Source: three-view drawing plus pictorial views. Frame: mm from the lowest corner of the part. A direction names the side the tool comes from. Round coordinates to 2 decimals unless told otherwise and drop trailing zeros. Loops run counter-clockwise (first coordinate to the right, second up) from the corner with the lowest first, then second, coordinate; pieces in that order, holes last. Notation, with made-up numbers: (82, 23) -> (116, 23) arc R28 cw to (116, 46) -> close; hole circle Ø8 at (-10, 59.5). An arc over 180 degrees is marked (long way). Return JSON: item names as keys, results as strings. Group by question number.
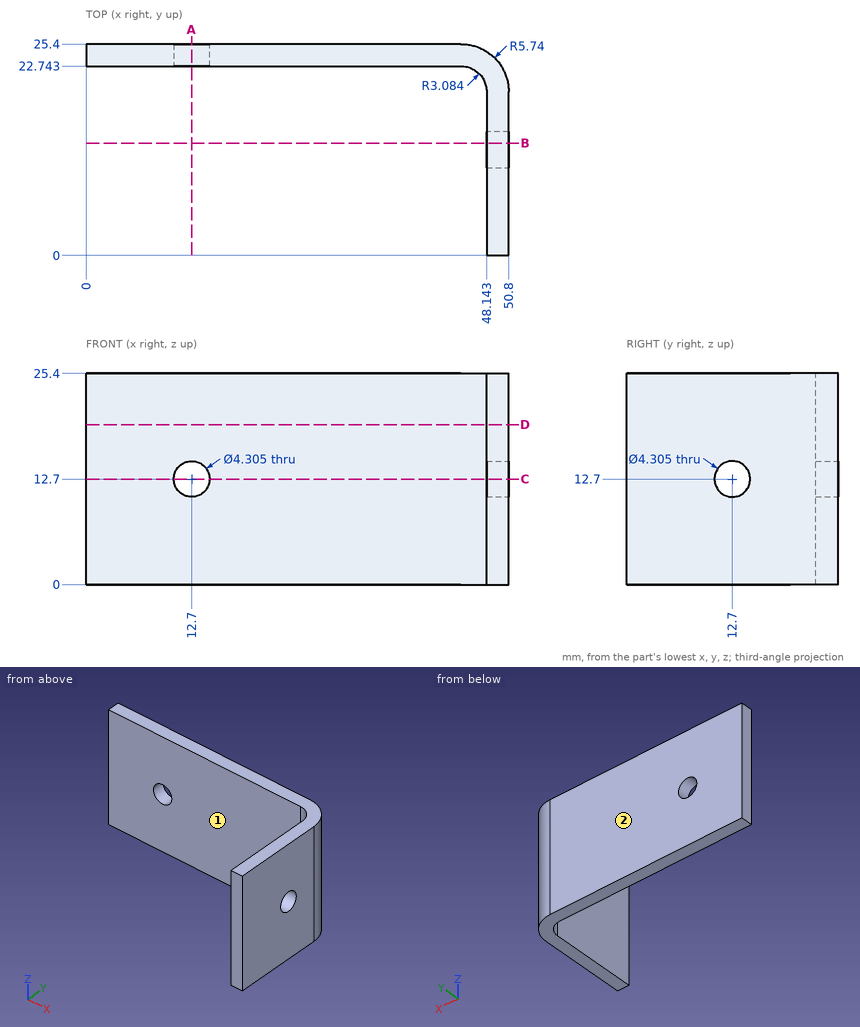
(1) Cut plane A-A (x = 12.7). Return loops of the section in (y, z).
(2) Cut plane C-C (z = 12.7). Return loops of the section in (x, y).
(3) Pin query (flat end, axial travel): pin 1 (5 mm diameter, centred on x = 12.7, z = 12.7, fed in from +Y); pin 2 (12 mm diameter, centred on x = 18, z = 19, fed in from -Y); pin 3 (3 mm diameter, centred on y = 12, z = 13.5, fed in from -X); pin 4 (12 mm diameter, centred on y = 15.5, z = 20, fed in from -X) (1 decimal). Return the tip coordinate at first contact, or that it passes through.
(4) Cut plane B-B (y = 13.5). Return loops of the section in (x, z).
(5) Set-up query: the marked faces 1 and 2. Return all of +Z, -Z, +X, -X, +Y, -Y with unobstructed straight access to the full face (end or side cutting, diameter ignored); none if empty.
(6) Cut plane D-D (z = 19.25). Return loops of the section in (x, y), and give its area (3 significant figures).
(7) Ray query, line 1 (Z direction, x = 49.95, y = 12.7); line 2 (Y direction, x = 15.5, z = 3.25); line 3 (X direction, y = 15.75, z = 23.5). Return the intervals inside material, ascending.
Answers follow:
{
 "1": {"outline": "(22.74, 0) -> (25.4, 0) -> (25.4, 10.55) -> (22.74, 10.55) -> close; (22.74, 14.85) -> (25.4, 14.85) -> (25.4, 25.4) -> (22.74, 25.4) -> close"},
 "2": {"outline": "(0, 22.74) -> (10.55, 22.74) -> (10.55, 25.4) -> (0, 25.4) -> close; (14.85, 22.74) -> (45.06, 22.74) arc R3.08 cw to (48.14, 19.66) -> (48.14, 14.85) -> (50.8, 14.85) -> (50.8, 19.66) arc R5.74 ccw to (45.06, 25.4) -> (14.85, 25.4) -> close; (48.14, 0) -> (50.8, 0) -> (50.8, 10.55) -> (48.14, 10.55) -> close"},
 "3": {"pin 1": "y = 25.4", "pin 2": "y = 22.74", "pin 3": "x = 48.14", "pin 4": "x = 47.5"},
 "4": {"outline": "(48.14, 0) -> (50.8, 0) -> (50.8, 10.7) -> (48.14, 10.7) -> close; (48.14, 14.7) -> (50.8, 14.7) -> (50.8, 25.4) -> (48.14, 25.4) -> close"},
 "5": {"face 1": "+Z, -Z, -X, -Y", "face 2": "+Z, -Z, +X, -X, +Y"},
 "6": {"outline": "(0, 22.74) -> (45.06, 22.74) arc R3.08 cw to (48.14, 19.66) -> (48.14, 0) -> (50.8, 0) -> (50.8, 19.66) arc R5.74 ccw to (45.06, 25.4) -> (0, 25.4) -> close", "area": "190 mm^2"},
 "7": {"line 1": "0 to 10.55, 14.85 to 25.4", "line 2": "22.74 to 25.4", "line 3": "48.14 to 50.8"}
}
